Geometry check sheet. Reference: the model listing, model coordinates, mm. Round coordinates to 2 decimals unless told otherwise and drop trailing zeros. Write each loop counter-clockwise with the first axis right and the second up, starting at its lowest first coordinate (ties: lowest second). Pieces come first, ordered by that corner, then holes. Notation, with made-up numbers: (-14.5, 77) - (33.5, 77) arc R28 ccw to (33.5, 112) - close; hole circle Ø3 at (54.25, 56.5). An arc over 180 degrees is marked (long way). Return JSON: item names as keys, results as strings. Group by question number.
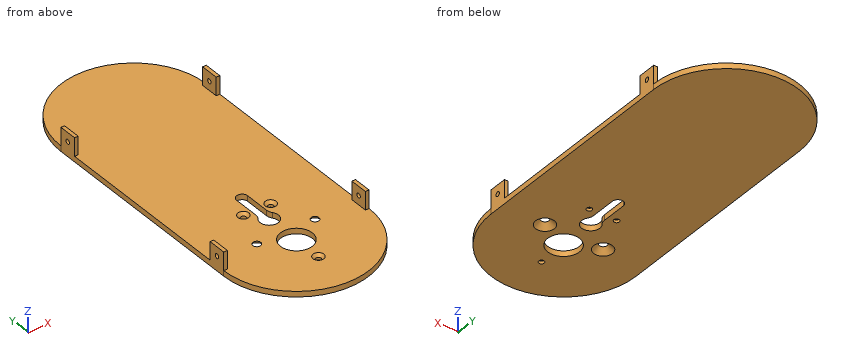
from build123d import *

# Parameters (mm, degrees)
SKETCH3_R           = 40
BOSS_EXTRUDE4_DEPTH = 3
SKETCH6_R           = 1.5
SKETCH6_R_2         = 8.75
CUT_EXTRUDE2_DEPTH  = 165.951508026
CHAMFER1_SIZE       = 1.5
SKETCH12_W          = 2
SKETCH12_H          = 10
BOSS_EXTRUDE7_DEPTH = 10
SKETCH13_R          = 1.25
CUT_EXTRUDE8_DEPTH  = 180.357185527
SKETCH14_R          = 2.15
CUT_EXTRUDE9_DEPTH  = 166.435788148
CHAMFER2_SIZE       = 3
CUT_EXTRUDE10_DEPTH = 166.435788148
FILLET1_R           = 5


with BuildPart() as part:
    # Sketch3 → Boss-Extrude4 (new body)
    with BuildSketch(Plane.XY):
        with BuildLine():
            ThreePointArc((40, 0), (0, 40), (-40, 0))
            Line((-40, 0), (40, 0))
        make_face()
        with BuildLine():
            Line((40, 0), (-40, 0))
            ThreePointArc((-40, 0), (0, -40), (40, 0))
        make_face()
        with BuildLine():
            Line((-40, 120), (-40, 0))
            ThreePointArc((-40, 0), (0, 40), (40, 0))
            Line((40, 0), (40, 120))
            ThreePointArc((40, 120), (0, 80), (-40, 120))
        make_face()
        with Locations((0, 120)):
            Circle(SKETCH3_R)
    extrude(amount=BOSS_EXTRUDE4_DEPTH)

    # Sketch6 → Cut-Extrude2 (cut, through all)
    with BuildSketch(Plane(origin=(0, 0, 0), x_dir=(-1, 0, 0), z_dir=(0, 0, -1))):
        with Locations((-7.5, 29.007101127)):
            Circle(SKETCH6_R)
        with Locations((7.5, 29.007101127)):
            Circle(SKETCH6_R)
        with Locations((0, -16.25)):
            Circle(SKETCH6_R)
        Circle(SKETCH6_R_2)
    extrude(amount=-CUT_EXTRUDE2_DEPTH, mode=Mode.SUBTRACT)

    # Chamfer1
    chamfer1_edges = [part.edges().sort_by_distance(p)[0] for p in [
        (-6, 29.007101127, 3),
        (1.5, -16.25, 3),
        (9, 29.007101127, 3),
    ]]
    chamfer(chamfer1_edges, length=CHAMFER1_SIZE)

    # Sketch12 → Boss-Extrude7 (add)
    with BuildSketch(Plane.XY.offset(3)):
        with Locations((39, 115)):
            Rectangle(SKETCH12_W, SKETCH12_H)
        with Locations((-39, 115)):
            Rectangle(SKETCH12_W, SKETCH12_H)
        with Locations((-39, 5)):
            Rectangle(SKETCH12_W, SKETCH12_H)
        with Locations((39, 5)):
            Rectangle(SKETCH12_W, SKETCH12_H)
    extrude(amount=BOSS_EXTRUDE7_DEPTH)

    # Sketch13 → Cut-Extrude8 (cut, through all)
    with BuildSketch(Plane.ZY.offset(40)):
        with Locations((8, 115)):
            Circle(SKETCH13_R)
        with Locations((8, 5)):
            Circle(SKETCH13_R)
    extrude(amount=-CUT_EXTRUDE8_DEPTH, mode=Mode.SUBTRACT)

    # Sketch14 → Cut-Extrude9 (cut, through all)
    with BuildSketch(Plane(origin=(0, 0, 0), x_dir=(-1, 0, 0), z_dir=(0, 0, -1))):
        with Locations((-16, 7.7)):
            Circle(SKETCH14_R)
        with Locations((16, 7.7)):
            Circle(SKETCH14_R)
    extrude(amount=-CUT_EXTRUDE9_DEPTH, mode=Mode.SUBTRACT)

    # Chamfer2
    chamfer2_edges = [part.edges().sort_by_distance(p)[0] for p in [
        (18.15, 7.7, 0),
        (-13.85, 7.7, 0),
    ]]
    chamfer(chamfer2_edges, length=CHAMFER2_SIZE - 0.0001)  # a hair under: the kernel refuses the full size

    # Sketch9 → Cut-Extrude10 (cut, through all)
    with BuildSketch(Plane(origin=(0, 0, 0), x_dir=(-1, 0, 0), z_dir=(0, 0, -1))):
        with BuildLine():
            ThreePointArc((3, 40), (0, 43), (-3, 40))
            Line((-3, 40), (-3, 24))
            ThreePointArc((-3, 24), (0, 15), (3, 24))
            Line((3, 24), (3, 40))
        make_face()
    extrude(amount=-CUT_EXTRUDE10_DEPTH, mode=Mode.SUBTRACT)

    # Fillet1
    fillet1_edges = [part.edges().sort_by_distance(p)[0] for p in [
        (3, 24, 1.5),
        (-3, 24, 1.5),
    ]]
    fillet(fillet1_edges, radius=FILLET1_R)


solid = part.part
1. Section check A-A (y = 20.5). Enter the section's corners in (x, z).
2. Depth check by flat-ended pin: pin 1 Ø1 at (x, z) = (39.5, 10) entering from +Y; pin 2 Ø5 at (x, y) = (-14.5, 97) entering from +Z; pin 3 Ø1.6 at (x, z) = (-39, 7.5) entering from -Y. Enter the tip coordinate at first touch or a pass-through.
3. Material ranges on line 1 along Y through (x, z) = (-38.9, 8); line 2 along X through (y, z) = (116.5, 7.75); line 3 along X through (y, z) = (20, 1.2), recorded low to high.
4. Section check D-D (y = 55.5). Enter the section's corners in (x, z).
5. Section check C-C (y = -2). Enter the section's corners in (x, z), and give its area (3 significant figures).
Result sheet:
{
 "1": {"outline": "(-40, 0) - (-4.97, 0) - (-4.97, 3) - (-40, 3) - close; (4.97, 0) - (40, 0) - (40, 3) - (4.97, 3) - close"},
 "2": {"pin 1": "stops at y = 120", "pin 2": "stops at z = 3", "pin 3": "stops at y = 0"},
 "3": {"line 1": "y = 0 to 3.75, 6.25 to 10, 110 to 113.75, 116.25 to 120", "line 2": "x = -40 to -38, 38 to 40", "line 3": "x = -40 to -5, 5 to 40"},
 "4": {"outline": "(-40, 0) - (40, 0) - (40, 3) - (-40, 3) - close"},
 "5": {"outline": "(-39.95, 0) - (-8.52, 0) - (-8.52, 3) - (-39.95, 3) - close; (8.52, 0) - (39.95, 0) - (39.95, 3) - (8.52, 3) - close", "area": "189 mm²"}
}
